For this review, take the finished solid that the model builds, in its own axes (mm). Round coordinates to 2 decimals unless told otherwise and drop trailing zeros. Order: outer loops, then holes, each group sorted by start corner. A loop starts at its lowest first (then second) coordinate and runs counter-clockwise, first axis right, second up. Notation, with made-up numbers: (12.25, 78.5) -> (61.25, 78.5) arc R3 ccw to (61.25, 83.5) -> close; hole circle Ø10 at (-23, -4.75). An arc over 180 degrees is marked (long way). Use a Markdown table: item, result. Add a question column.
1) Consider section A-A (x = -33). State the section outline as (y, z) points (3 decimals).
2) Consider section B-B (y = 12.7). State the section outline as (x, z) points (3 decimals), plus the area to 3 significant figures.
3) Wall thickness on line 1 along Y through (x, z) = (12.7, 1.7); line 2 along Y through (x, z) = (-50.5, 0.2); line 3 along X through (y, z) = (97.5, 2.25): over which ranges is each line inside the solid? List them lowest first. Write a range as [from, to].
4) Consider section D-D (z = 0.5). Give the number of separate pieces and of enclosed holes in the cut face, plus the area to 3 significant figures.
5) Clearance check with flat-ended pins moving along their axes: P1, Ø1.6, axis at x = -26.5, z = 2, coming from the -Y side; P2, Ø1.6, axis at y = 130.5, z = 2, coming from the -X side; P3, Ø1.6, axis at x = -39, z = 2.5, coming from the +Y side. State where each tip first meets the part, or that it passes through.
6) Consider section C-C (y = 43). State the section outline as (x, z) points (3 decimals), plus the area to 3 significant figures.
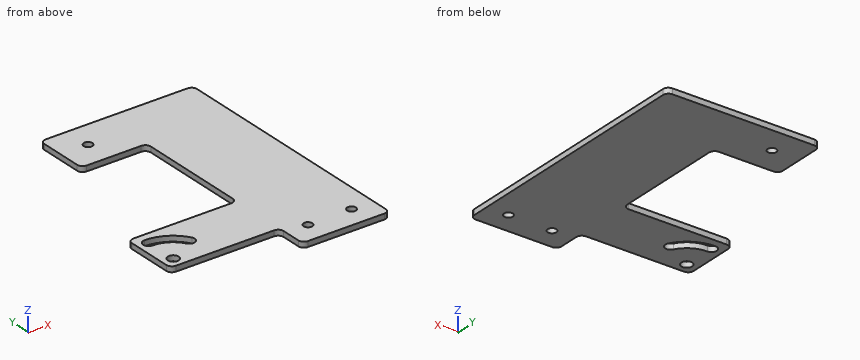
```python
from build123d import *

# Parameters (mm, degrees)
SKETCH1_W           = 50.8
SKETCH1_H           = 50.8
SKETCH1_R           = 2.5527
SKETCH1_W_2         = 63.5
SKETCH1_H_2         = 33.02
SKETCH1_R_2         = 3.175
BOSS_EXTRUDE1_DEPTH = 3.175
SKETCH1_4_W         = 50.8
SKETCH1_4_H         = 101.6
SKETCH1_4_W_2       = 38.1
SKETCH1_4_H_2       = 31.75
BOSS_EXTRUDE2_DEPTH = 3.175
FILLET1_R           = 3.175
SKETCH2_R           = 2.5527
CUT_EXTRUDE1_DEPTH  = 25.4


with BuildPart() as part:
    # Sketch1 → Boss-Extrude1 (new body)
    # profile 1 of 2: a face of its own
    with BuildSketch(Plane.XY):
        with Locations((25.4, 25.4)):
            Rectangle(SKETCH1_W, SKETCH1_H)
        with Locations((38.1, 12.7)):
            Circle(SKETCH1_R, mode=Mode.SUBTRACT)
        with Locations((12.7, 12.7)):
            Circle(SKETCH1_R, mode=Mode.SUBTRACT)
    # profile 2 of 2: a face of its own
    with BuildSketch(Plane.XY):
        with Locations((-31.75, 34.29)):
            Rectangle(SKETCH1_W_2, SKETCH1_H_2)
        with Locations((-57.15, 24.13)):
            Circle(SKETCH1_R_2, mode=Mode.SUBTRACT)
        with BuildLine():
            ThreePointArc((-57.15, 46.355), (-46.0375, 43.377414599), (-37.902585401, 35.2425))
            ThreePointArc((-37.902585401, 35.2425), (-39.064716058, 30.905369343), (-43.401846715, 32.0675))
            ThreePointArc((-43.401846715, 32.0675), (-49.2125, 37.878153285), (-57.15, 40.005))
            ThreePointArc((-57.15, 40.005), (-60.325, 43.18), (-57.15, 46.355))
        make_face(mode=Mode.SUBTRACT)
    extrude(amount=BOSS_EXTRUDE1_DEPTH)

    # Sketch1_4 → Boss-Extrude2 (add)
    with BuildSketch(Plane.XY):
        with Locations((25.4, 101.6)):
            Rectangle(SKETCH1_4_W, SKETCH1_4_H)
        with Locations((-19.05, 136.525)):
            Rectangle(SKETCH1_4_W_2, SKETCH1_4_H_2)
    extrude(amount=BOSS_EXTRUDE2_DEPTH)

    # Fillet1
    fillet1_edges = [part.edges().sort_by_distance(p)[0] for p in [
        (0, 0, 1.5875),
        (0, 17.78, 1.5875),
        (-63.5, 17.78, 1.5875),
        (-63.5, 50.8, 1.5875),
        (50.8, 0, 1.5875),
        (0, 50.8, 1.5875),
        (50.8, 152.4, 1.5875),
        (-38.1, 152.4, 1.5875),
        (-38.1, 120.65, 1.5875),
        (0, 120.65, 1.5875),
    ]]
    fillet(fillet1_edges, radius=FILLET1_R)

    # Sketch2 → Cut-Extrude1 (cut)
    with BuildSketch(Plane.XY.offset(3.175)):
        with Locations((-22.225, 136.525)):
            Circle(SKETCH2_R)
    extrude(amount=-CUT_EXTRUDE1_DEPTH, mode=Mode.SUBTRACT)


solid = part.part
```
Results list:
| question | item | result |
|---|---|---|
| 1 | outline | (17.78, 0) -> (50.8, 0) -> (50.8, 3.175) -> (17.78, 3.175) -> close; (120.65, 0) -> (152.4, 0) -> (152.4, 3.175) -> (120.65, 3.175) -> close |
| 2 | outline | (0, 0) -> (10.147, 0) -> (10.147, 3.175) -> (0, 3.175) -> close; (15.253, 0) -> (35.547, 0) -> (35.547, 3.175) -> (15.253, 3.175) -> close; (40.653, 0) -> (50.8, 0) -> (50.8, 3.175) -> (40.653, 3.175) -> close |
| 2 | area | 129 mm2 |
| 3 | line 1 | [0, 10.15], [15.25, 152.4] |
| 3 | line 2 | [17.78, 38.55], [45.34, 50.8] |
| 3 | line 3 | [0, 50.8] |
| 4 | separate pieces | 1 |
| 4 | enclosed holes | 5 |
| 4 | area | 10,800 mm2 |
| 5 | P1 | y = 17.78 |
| 5 | P2 | x = -38.1 |
| 5 | P3 | y = 50.8 |
| 6 | outline | (-63.5, 0) -> (-60.32, 0) -> (-60.32, 3.175) -> (-63.5, 3.175) -> close; (-45.408, 0) -> (50.8, 0) -> (50.8, 3.175) -> (-45.408, 3.175) -> close |
| 6 | area | 316 mm2 |
